```python
from build123d import *

# Parameters (mm, degrees)
BOSS_EXTRUDE2_DEPTH = 38.1
CUT_EXTRUDE1_REACH  = 383


with BuildPart() as part:
    # Sketch1 → Boss-Extrude2 (new body)
    with BuildSketch(Plane(origin=(0, 0, 0), x_dir=(0, 0, -1), z_dir=(1, 0, 0))):
        Polygon((230.790126839, 0), (446.057536726, 140.777827649), (446.057536726, 381), (263.652, 381), (263.652, 190.5), (0, 190.5), (0, 0), align=None)
    extrude(amount=BOSS_EXTRUDE2_DEPTH)

    # Sketch2 → Cut-Extrude1 (cut, up to next)
    with BuildSketch(Plane(origin=(0, 381, 0), x_dir=(1, 0, 0), z_dir=(0, 1, 0)), mode=Mode.PRIVATE) as cut_extrude1_sk1:
        Polygon((38.1, 446.057536726), (0, 407.957536726), (0, 446.057536726), align=None)
    cut_extrude1_tool1 = extrude(cut_extrude1_sk1.sketch, amount=-CUT_EXTRUDE1_REACH, mode=Mode.PRIVATE) & part.part
    add(cut_extrude1_tool1.solids().sort_by_distance((12.7, 381, -433.357537))[0], mode=Mode.SUBTRACT)


solid = part.part
```
For this review, take the finished solid that the model builds, in its own axes (mm). A direction names the side the tool comes from. Coordinates: 2 decimals unless noted, no trailing zeros. Loops run counter-clockwise (first coordinate to the right, second up) from the corner with the lowest first, then second, coordinate; pieces in that order, holes last.
1. Add section C-C, the plane y = 146.5. Give the boundary of the cut face in (x, z).
2. For line 1 (Y direction, x = 16, z = -50); line 2 (Y direction, x = 4, z = -345); line 3 (Z direction, x = 9.5, y = 326), list the stretches that pass through material, from the lowest coordinate up.
3. Add section B-B, the plane z = -158. Give the boundary of the cut face in (x, y), then the cut area to 3 significant figures.
4. Insertion check: P1, Ø2, axis at x = 26, y = 297.5, coming from the -Z side; P2, Ø1, axis at x = 15, z = -289, coming from the -Y side; P3, Ø6, axis at x = 17.5, y = 319.5, coming from the -Z side. Each pin has a flat end and moves straight along its axis. Give the tip position at first contact, or say it passes through.
5. Add section A-A, the plane x = 14. Give the boundary of the cut face in (y, z).
6. For faces 1 (the flat face through (19, 381, -356)), 2 (the flat face through (19, 190.5, -134)), list the 3-axis set-ups (+Z, -Z, +X, -X, +Y, -Y) from which the entire face can be reached by the end or side of a thin tool; tool diameter is ignored.
Result:
1. outline: (0, -407.96) - (38.1, -446.06) - (38.1, 0) - (0, 0) - close
2. line 1: y = 0 to 190.5
2. line 2: y = 74.69 to 381
2. line 3: z = -417.46 to -263.65
3. outline: (0, 0) - (38.1, 0) - (38.1, 190.5) - (0, 190.5) - close
3. area: 7,260 mm2
4. P1: stops at z = -434.96
4. P2: stops at y = 37.74
4. P3: stops at z = -428.46
5. outline: (0, -230.79) - (125.02, -421.96) - (381, -421.96) - (381, -263.65) - (190.5, -263.65) - (190.5, 0) - (0, 0) - close
6. face 1: +Z, -Z, +X, -X, +Y
6. face 2: +Z, +X, -X, +Y
